Read the model definition and answer for the solid it produces. Units are mm, in the model's axes. A direction names the side the tool comes from. Coordinates: 2 decimals unless noted, no trailing zeros. Order: outer loops, then holes, each group sorted by start corner. A loop starts at its lowest first (then second) coordinate and runs counter-clockwise, first axis right, second up. Notation, with made-up numbers: (19, 20.25) -> (47, 20.25) arc R23 ccw to (47, 30.25) -> close; hole circle Ø3 at (80.5, 64). An arc over 180 degrees is marked (long way). Answer in a Markdown table with one row per item.
from build123d import *

# Parameters (mm, degrees)
F1_DEPTH = 9.525
F3_DEPTH = 6.35
F5_DEPTH = 3.175


with BuildPart() as f1:
    # F0 (on Front) → F1 (new body)
    with BuildSketch(Plane.XZ):
        with BuildLine():
            ThreePointArc((63.5, 95.25), (61.640128, 99.740128), (57.15, 101.6))
            Line((57.15, 101.6), (-57.15, 101.6))
            ThreePointArc((-57.15, 101.6), (-61.640128, 99.740128), (-63.5, 95.25))
            Line((-63.5, 95.25), (-63.5, -95.25))
            ThreePointArc((-63.5, -95.25), (-61.640128, -99.740128), (-57.15, -101.6))
            Line((-57.15, -101.6), (57.15, -101.6))
            ThreePointArc((57.15, -101.6), (61.640128, -99.740128), (63.5, -95.25))
            Line((63.5, -95.25), (63.5, 95.25))
        make_face()
    extrude(amount=F1_DEPTH)

    # F2 (on face) → F3 (cut)
    with BuildSketch(Plane.XZ.offset(9.525)):
        with BuildLine():
            ThreePointArc((60.325, 95.25), (59.395064, 97.495064), (57.15, 98.425))
            Line((57.15, 98.425), (-57.15, 98.425))
            ThreePointArc((-57.15, 98.425), (-59.395064, 97.495064), (-60.325, 95.25))
            Line((-60.325, 95.25), (-60.325, -95.25))
            ThreePointArc((-60.325, -95.25), (-59.395064, -97.495064), (-57.15, -98.425))
            Line((-57.15, -98.425), (57.15, -98.425))
            ThreePointArc((57.15, -98.425), (59.395064, -97.495064), (60.325, -95.25))
            Line((60.325, -95.25), (60.325, 95.25))
        make_face()
    extrude(amount=-F3_DEPTH, mode=Mode.SUBTRACT)

    # F4 (on face) → F5 (cut, through all)
    with BuildSketch(Plane.XZ.offset(3.175)):
        with BuildLine():
            ThreePointArc((31.129177, 69.260782), (35.227664, 63.396759), (39.326151, 69.260782))
            ThreePointArc((39.326151, 69.260782), (35.227664, 80.46103), (31.129177, 69.260782))
        make_face()
    extrude(amount=-F5_DEPTH, mode=Mode.SUBTRACT)


solid = f1.part
Q1. Given pin 1 (14 mm diameter, centred on x = 35.23, z = 67.76, fed in from -Y) (3 decimals), flat-ended and moving along its own axis, determine where the tip first touches the part or whether it passes through.
Outcome:
| item | result |
|---|---|
| pin 1 | y = -3.175 |
Q2. The part is cut by section A-A (x = -48.5). Write down the section's boundary in (y, z) (3 decimals).
Outcome:
| item | result |
|---|---|
| outline | (-9.525, -101.6) -> (0, -101.6) -> (0, 101.6) -> (-9.525, 101.6) -> (-9.525, 98.425) -> (-3.175, 98.425) -> (-3.175, -98.425) -> (-9.525, -98.425) -> close |
Q3. For a pull along X with two mould halves and no side action, classify faces 3 (the face through (35.1, -1.6, 63.4)), 4 (the face through (61.59, -4.7, -99.79)), 5 (the face through (-1, -5, -101.6)) as pulls with the +X half, pulls with the -X half, needs draft (parallel to the pull), parting line crosses it, or undercut.
Outcome:
| item | result |
|---|---|
| face 3 | undercut |
| face 4 | pulls with the +X half |
| face 5 | needs draft |
Q4. The part is cut by section C-C (z = 48). Write down the section's boundary in (x, y) (3 decimals), then the cut area to 3 significant figures.
Outcome:
| item | result |
|---|---|
| outline | (-63.5, -9.525) -> (-60.325, -9.525) -> (-60.325, -3.175) -> (60.325, -3.175) -> (60.325, -9.525) -> (63.5, -9.525) -> (63.5, 0) -> (-63.5, 0) -> close |
| area | 444 mm² |
Q5. For faces 1 (the face through (63.5, -5, -1)), 2 (the face through (-60.325, -6, 1)), determine the directions among +Z, -Z, +X, -X, +Y, -Y from which every point of the face is accessible in a straight line to the end or side of a thin tool.
Outcome:
| item | result |
|---|---|
| face 1 | +Z, -Z, +X, +Y, -Y |
| face 2 | -Y |
Q6. The part is cut by section B-B (y = -5.5). Write down the section's boundary in (x, z) (3 decimals).
Outcome:
| item | result |
|---|---|
| outline | (-63.5, -95.25) arc R6.35 ccw to (-57.15, -101.6) -> (57.15, -101.6) arc R6.35 ccw to (63.5, -95.25) -> (63.5, 95.25) arc R6.35 ccw to (57.15, 101.6) -> (-57.15, 101.6) arc R6.35 ccw to (-63.5, 95.25) -> close; hole (-60.325, -95.25) arc R3.175 ccw to (-57.15, -98.425) -> (57.15, -98.425) arc R3.175 ccw to (60.325, -95.25) -> (60.325, 95.25) arc R3.175 ccw to (57.15, 98.425) -> (-57.15, 98.425) arc R3.175 ccw to (-60.325, 95.25) -> close |
Q7. Consider line 1 (Z direction, x = 7, y = -3.25) (3 decimals); line 2 (X direction, y = -3.5, z = 82) (3 decimals); line 3 (Y direction, x = -30, z = 2) (3 decimals). Determine where each line is inside the solid, lowest interval first.
Outcome:
| item | result |
|---|---|
| line 1 | -101.6 to -98.425, 98.425 to 101.6 |
| line 2 | -63.5 to -60.325, 60.325 to 63.5 |
| line 3 | -3.175 to 0 |
